from build123d import *

# Parameters (mm, degrees)
EXTRUDE_1_DEPTH        = 300
SKETCH_2_R             = 3
SKETCH_2_R_2           = 1.75
CUT_EXTRUDE_1_DEPTH    = 4.5
SKETCH_2_2_R           = 1.75
CUT_EXTRUDE_2_DEPTH    = 9
PATTERN_LINEAR_1_COUNT = 12
PATTERN_LINEAR_1_PITCH = 25


with BuildPart() as part:
    # Эскиз1 → Бобышка-Вытянуть1 (new body)
    with BuildSketch(Plane.XY):
        with BuildLine():
            Line((-6, 3.7), (-5.7, 4))
            Line((-5.7, 4), (5.7, 4))
            Line((5.7, 4), (6, 3.7))
            Line((6, 3.7), (6, 2.449776022))
            ThreePointArc((6, 2.449776022), (5.561887715, 2.168810579), (5.297911886, 1.720256551))
            Line((5.297911886, 1.720256551), (4.687472904, 1.720256551))
            Line((4.687472904, 1.720256551), (4.687472904, 1.082255421))
            Line((4.687472904, 1.082255421), (5.292171789, 1.082255421))
            ThreePointArc((5.292171789, 1.082255421), (5.554928022, 0.621665058), (6, 0.333402583))
            Line((6, 0.333402583), (6, -3.7))
            Line((6, -3.7), (5.7, -4))
            Line((5.7, -4), (-5.7, -4))
            Line((-5.7, -4), (-6, -3.7))
            Line((-6, -3.7), (-6, 0.333402583))
            ThreePointArc((-6, 0.333402583), (-5.554928022, 0.621665058), (-5.292171789, 1.082255421))
            Line((-5.292171789, 1.082255421), (-4.687472904, 1.082255421))
            Line((-4.687472904, 1.082255421), (-4.687472904, 1.720256551))
            Line((-4.687472904, 1.720256551), (-5.297911886, 1.720256551))
            ThreePointArc((-5.297911886, 1.720256551), (-5.561887715, 2.168810579), (-6, 2.449776022))
            Line((-6, 2.449776022), (-6, 3.7))
        make_face()
    extrude(amount=EXTRUDE_1_DEPTH)

    # Эскиз2 → Вырез-Вытянуть1 (cut)
    with BuildSketch(Plane(origin=(0, 4, 0), x_dir=(1, 0, 0), z_dir=(0, 1, 0))):
        with Locations((0.188190244, -10)):
            Circle(SKETCH_2_R)
        with Locations((0.188190244, -10)):
            Circle(SKETCH_2_R_2, mode=Mode.SUBTRACT)
    cut_extrude_1 = extrude(amount=-CUT_EXTRUDE_1_DEPTH, mode=Mode.SUBTRACT)

    # Эскиз2<2> → Вырез-Вытянуть2 (cut, through all)
    with BuildSketch(Plane(origin=(0, 4, 0), x_dir=(1, 0, 0), z_dir=(0, 1, 0))):
        with Locations((0.188190244, -10)):
            Circle(SKETCH_2_2_R)
    cut_extrude_2 = extrude(amount=-CUT_EXTRUDE_2_DEPTH, mode=Mode.SUBTRACT)

    # Линейный массив1: Вырез-Вытянуть1, Вырез-Вытянуть2 ×12
    with Locations(*[(0, 0, i * PATTERN_LINEAR_1_PITCH) for i in range(1, PATTERN_LINEAR_1_COUNT)]):
        add(cut_extrude_1, mode=Mode.SUBTRACT)
        add(cut_extrude_2, mode=Mode.SUBTRACT)


solid = part.part
For this review, take the finished solid that the model builds, in its own axes (mm). A direction names the side the tool comes from. Round coordinates to 2 decimals unless told otherwise and drop trailing zeros. Order: outer loops, then holes, each group sorted by start corner. A loop starts at its lowest first (then second) coordinate and runs counter-clockwise, first axis right, second up. Notation, with made-up numbers: (38.25, 72.5) -> (62.25, 72.5) arc R28 ccw to (62.25, 108.5) -> close; hole circle Ø1 at (55.25, 56.5). An arc over 180 degrees is marked (long way). Write item = value, one per line. Start each with the question number.
1) Insertion check: pin 1 (5 mm diameter, centred on x = 0.5, z = 210, fed in from +Y). The pin has a flat end and moves straight along its axis. Give the tip position at first contact, or say it passes through.
2) Tool access review of faces 3 (the face through (0, -4, 148)), 4 (the face through (-0.46, 1.78, 87.93)): name each direction out of +Z, -Z, +X, -X, +Y, -Y from which nothing blocks a thin tool from reaching the whole face with its end or side.
3) Take a section at A-A on z = 149. State the section outline as (x, y) points, plus the area to 3 significant figures.
4) To check wall thickness, follow line 1 (X direction, y = -2.8, z = 260); line 2 (Y direction, x = 0, z = 83); line 3 (X direction, y = 1.95, z = 60). State the ranges of each line that lie inside material, in increasing order. Write a range as from..to.
5) The part is to be moulded in two halves that separate along X. For faces 1 (the face through (0, 4, 148)), 2 (the face through (0, -0.5, 12)), say which applies: +X half, -X half, draft (parallel to the pull), parting line (faces both ways), or undercut.
Verdict:
q1.pin_1 = -0.5
q2.face_3 = +Z, -Z, +X, -X, -Y
q2.face_4 = +Y
q3.outline = (-6, -3.7) -> (-5.7, -4) -> (5.7, -4) -> (6, -3.7) -> (6, 0.33) arc R1.12 cw to (5.29, 1.08) -> (4.69, 1.08) -> (4.69, 1.72) -> (5.3, 1.72) arc R1.12 cw to (6, 2.45) -> (6, 3.7) -> (5.7, 4) -> (-5.7, 4) -> (-6, 3.7) -> (-6, 2.45) arc R1.12 cw to (-5.3, 1.72) -> (-4.69, 1.72) -> (-4.69, 1.08) -> (-5.29, 1.08) arc R1.12 cw to (-6, 0.33) -> close
q3.area = 92.8 mm2
q4.line_1 = -6..-1.56, 1.94..6
q4.line_2 = -4..-0.5
q4.line_3 = -5.4..-2.81, 3.19..5.4
q5.face_1 = draft
q5.face_2 = undercut
